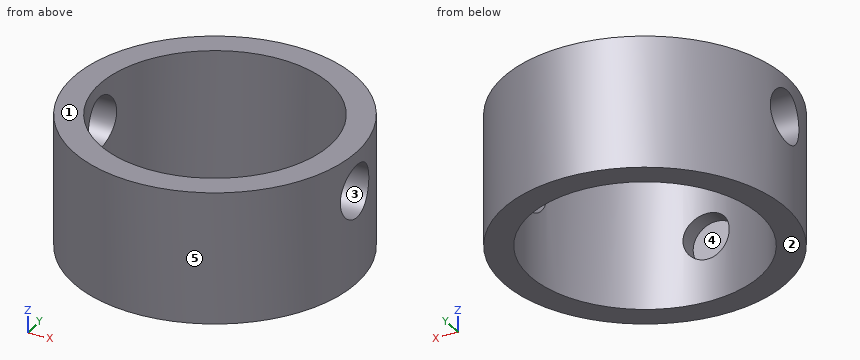
from build123d import *

# Parameters (mm, degrees)
ESQUISSE1_R             = 10.75
ESQUISSE1_R_2           = 8.75
BOSS_EXTRU_1_DEPTH      = 10
ESQUISSE2_R             = 1.75
ENL_V_MAT_EXTRU_1_DEPTH = 10
ESQUISSE3_R             = 2
ENL_V_MAT_EXTRU_2_DEPTH = 15


with BuildPart() as part:
    # Esquisse1 → Boss.-Extru.1 (new body)
    with BuildSketch(Plane.XY):
        Circle(ESQUISSE1_R)
        Circle(ESQUISSE1_R_2, mode=Mode.SUBTRACT)
    extrude(amount=BOSS_EXTRU_1_DEPTH)

    # Esquisse2 → Enlèv. mat.-Extru.1 (cut)
    with BuildSketch(Plane(origin=(0, 0, 0), x_dir=(1, 0, 0), z_dir=(0, 1, 0))):
        with Locations((0, -5)):
            Circle(ESQUISSE2_R)
    extrude(amount=-ENL_V_MAT_EXTRU_1_DEPTH, mode=Mode.SUBTRACT)

    # Esquisse3 → Enlèv. mat.-Extru.2 (cut, symmetric)
    with BuildSketch(Plane(origin=(0, 0, 0), x_dir=(0, 0, -1), z_dir=(1, 0, 0))):
        with Locations((-7, 0)):
            Circle(ESQUISSE3_R)
    extrude(amount=ENL_V_MAT_EXTRU_2_DEPTH, both=True, mode=Mode.SUBTRACT)


solid = part.part
Model file for the job. Use its own axes, mm. Face numbers are marked on the shaded views. A direction names the side the tool comes from. Give positions to 0.01 mm unless a question says otherwise; leave off trailing zeros. Order: outer loops, then holes, each group sorted by start corner. A loop starts at its lowest first (then second) coordinate and runs counter-clockwise, first axis right, second up. Notation, with made-up numbers: M 67,44.5 L 85,44.5 A31 cw 85,73.5 Z; hole C 84,-12 d11. An arc over 180 degrees is marked long. Write item = value, one per line.
Q1. Tool access for the marked faces 4 and 5: list every direction of +Z, -Z, +X, -X, +Y, -Y with a clear straight run to the whole face (end or side of a thin tool).
Derived:
face_4 = none
face_5 = +Z, -Z
Q2. Drill centre lines: line 1 (Z direction, x = 0, y = -9.1); line 2 (Z direction, x = 9.1, y = 0); line 3 (X direction, y = 0, z = 3). Where is each one in solid material? Low to high. Write a range as [from, to].
Derived:
line_1 = [0, 3.25], [6.75, 10]
line_2 = [0, 5], [9, 10]
line_3 = [-10.75, -8.75], [8.75, 10.75]
Q3. Flat gauge pins, fed straight in: pin 1 (5 mm diameter, centred on y = 0, z = 7, fed in from +X); pin 2 (5 mm diameter, centred on x = -6.5, z = 5.5, fed in from +Y); pin 3 (3 mm diameter, centred on y = 7, z = 1.5, fed in from +X); pin 4 (6 mm diameter, centred on y = 3.5, z = 1.5, fed in from +X). Where does each tip first touch, or does it go through?
Derived:
pin_1 = 10.75
pin_2 = 9.98
pin_3 = 9.24
pin_4 = 10.74
Q4. Cut at C-C, the plane y = 8. List the corners of the cut face in (x, z), then the cut area to 3 significant figures.
Derived:
outline = M -7.18,0 L -3.54,0 L -3.54,10 L -7.18,10 Z; M 3.54,0 L 7.18,0 L 7.18,10 L 3.54,10 Z
area = 72.7 mm2
Q5. Cut at A-A, the plane y = 0. List the corners of the cut face in (x, z).
Derived:
outline = M -10.75,0 L -8.75,0 L -8.75,5 L -10.75,5 Z; M -10.75,9 L -8.75,9 L -8.75,10 L -10.75,10 Z; M 8.75,0 L 10.75,0 L 10.75,5 L 8.75,5 Z; M 8.75,9 L 10.75,9 L 10.75,10 L 8.75,10 Z
Q6. Two-plate mould, pull along Z, no slides. Class the marked faces 1, 2 and 3: pulls with the +Z half, pulls with the -Z half, needs draft (parallel to the pull), parting line crosses it, or undercut.
Derived:
face_1 = pulls with the +Z half
face_2 = pulls with the -Z half
face_3 = undercut
Q7. Cut at D-D, the plane z = 4.5. List the corners of the cut face in (x, y).
Derived:
outline = C 0,0 d21.5; hole M -1.68,-10 L 1.68,-10 L 1.68,-8.59 A8.75 ccw long -1.68,-8.59 Z
Q8. Cut at B-B, the plane x = 7.5. List the corners of the cut face in (y, z), then the cut area to 3 significant figures.
Derived:
outline = M -7.7,0 L -4.51,0 L -4.51,10 L -7.7,10 Z; M 4.51,0 L 7.7,0 L 7.7,10 L 4.51,10 Z
area = 63.9 mm2
